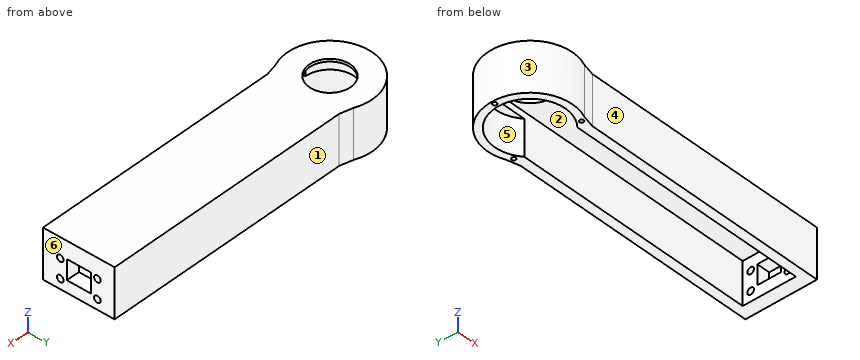
```python
from build123d import *

# Parameters (mm, degrees)
SKETCH025_R           = 32
PAD016_DEPTH          = 37
SKETCH026_R           = 18.5
POCKET001_DEPTH       = 35
SKETCH027_R           = 26.5
POCKET002_DEPTH       = 27
SKETCH028_R           = 15.5
POCKET003_DEPTH       = 37.001
PAD018_DEPTH          = 37
SKETCH034_W           = 40
SKETCH034_H           = 32
POCKET004_DEPTH       = 200
SKETCH046_W           = 54
SKETCH046_H           = 37
SKETCH046_W_2         = 18
SKETCH046_H_2         = 15
PAD020_DEPTH          = 10
SKETCH047_R           = 1.5
POCKET_DEPTH          = 10
POLARPATTERN003_COUNT = 3
CHAMFER002_SIZE       = 5
SKETCH063_R           = 2.5
POCKET022_DEPTH       = 10.001
BODY_PLACEMENT_ANGLE  = 179.999986


with BuildPart() as part:
    # Sketch025 (on Face1 of CopyPocket) → Pad016 (new body)
    with BuildSketch(Plane.XY.offset(19.5)):
        Circle(SKETCH025_R)
    extrude(amount=-PAD016_DEPTH)

    # Sketch026 (on Face3 of Pad016) → Pocket001 (cut)
    with BuildSketch(Plane(origin=(0, 0, -17.5), x_dir=(1, 0, 0), z_dir=(0, 0, -1))):
        Circle(SKETCH026_R)
    extrude(amount=-POCKET001_DEPTH, mode=Mode.SUBTRACT)

    # Sketch027 (on Face3 of Pocket001) → Pocket002 (cut)
    with BuildSketch(Plane(origin=(0, 0, -17.5), x_dir=(1, 0, 0), z_dir=(0, 0, -1))):
        Circle(SKETCH027_R)
    extrude(amount=-POCKET002_DEPTH, mode=Mode.SUBTRACT)

    # Sketch028 (on Face2 of Pocket002) → Pocket003 (cut, through all)
    with BuildSketch(Plane.XY.offset(19.5)):
        Circle(SKETCH028_R)
    extrude(amount=-POCKET003_DEPTH, mode=Mode.SUBTRACT)

    # Sketch030 (on Face2 of Pocket003) → Pad018 (join)
    with BuildSketch(Plane.XY.offset(19.5)):
        with BuildLine():
            ThreePointArc((-17.175564, 27), (-32, 0), (-17.175564, -27))
            Line((-200, -27), (-17.175564, -27))
            Line((-200, 27), (-200, -27))
            Line((-17.175564, 27), (-200, 27))
        make_face()
    extrude(amount=-PAD018_DEPTH)

    # Sketch034 (on Face2 of Pad018) → Pocket004 (cut)
    with BuildSketch(Plane(origin=(-200, 0, 0), x_dir=(0, -1, 0), z_dir=(-1, 0, 0))):
        with Locations((0, -1.5)):
            Rectangle(SKETCH034_W, SKETCH034_H)
    extrude(amount=-POCKET004_DEPTH, mode=Mode.SUBTRACT)

    # Sketch046 (on Face3 of Pocket004) → Pad020 (join)
    with BuildSketch(Plane(origin=(-200, 0, 0), x_dir=(0, -1, 0), z_dir=(-1, 0, 0))):
        with Locations((0, 1)):
            Rectangle(SKETCH046_W, SKETCH046_H)
        with Locations((0, -1)):
            Rectangle(SKETCH046_W_2, SKETCH046_H_2, mode=Mode.SUBTRACT)
    extrude(amount=PAD020_DEPTH)

    # Sketch047 (on Face20 of Pad020) → Pocket (cut)
    with BuildSketch(Plane(origin=(0, 0, -17.5), x_dir=(1, 0, 0), z_dir=(0, 0, -1))):
        with Locations((29.53, 0)):
            Circle(SKETCH047_R)
    pocket = extrude(amount=-POCKET_DEPTH, mode=Mode.SUBTRACT)

    # PolarPattern003: Pocket ×3 about axis
    polarpattern003_axis = Axis((0, 0, -17.5), (0, 0, -1))
    for i in range(1, POLARPATTERN003_COUNT):
        add(pocket.rotate(polarpattern003_axis, i * 360 / POLARPATTERN003_COUNT), mode=Mode.SUBTRACT)

    # Chamfer002
    chamfer002_edges = [part.edges().sort_by_distance(p)[0] for p in [
        (-17.175564, -27, 1),
        (-17.175564, 27, 1),
    ]]
    chamfer(chamfer002_edges, length=CHAMFER002_SIZE)

    # Sketch063 (on Face14 of Chamfer002) → Pocket022 (cut, through all)
    with BuildSketch(Plane.YZ.offset(-200)):
        with Locations((-14, 4.5)):
            Circle(SKETCH063_R)
        with Locations((14, 4.5)):
            Circle(SKETCH063_R)
        with Locations((-14, -10)):
            Circle(SKETCH063_R)
        with Locations((14, -10)):
            Circle(SKETCH063_R)
    extrude(amount=-POCKET022_DEPTH, mode=Mode.SUBTRACT)


with BuildPart() as part_1:
    # Body placement: moved
    add(part.part.moved(Location((5, -1e-06, 2.46221))).rotate(Axis((5, -1e-06, 2.46221), (0, 0, 1)), BODY_PLACEMENT_ANGLE))


solid = part_1.part
```
CAD build for the part. Positions are in the model's coordinates, mm. Face numbers are marked on the shaded views. A direction names the side the tool comes from. Give positions to 0.01 mm unless a question says otherwise; leave off trailing zeros. Write each loop counter-clockwise with the first axis right and the second up, starting at its lowest first coordinate (ties: lowest second). Pieces come first, ordered by that corner, then holes. Notation, with made-up numbers: M 54,57 L 113,57 A10 ccw 113,64 Z; hole C 54.5,-12 d3. An arc over 180 degrees is marked long. Return JSON: item names as keys, results as strings. Group by question number.
(1) Flat gauge pins, fed straight in: pin 1 Ø2 at (x, z) = (96.5, 14.5) entering from +Y; pin 2 Ø6 at (x, z) = (120.5, -7.5) entering from -Y; pin 3 Ø1.5 at (x, y) = (-24.5, 0.5) entering from -Z. Where does each tip first touch, or does it go through?
(2) 3-axis set-ups, long thin cutter, end or side, ignore diameter. For the marked faces 1, 2 and 3: which of +Z, -Z, +X, -X, +Y, -Y reach the whole face in a straight line?
(3) Mould opens along X. For the marked faces 4, 5 and 6 say: pulls with the +X half, pulls with the -X half, needs draft (parallel to the pull), parting line crosses it, or undercut.
(4) Band-saw the part on A-A (x = 103.5). Give the cut face in (y, z), and give its area (3 significant figures).
(5) Drill centre lines: L1, parallel to Y at x = 102.5, z = -8; L2, parallel to Y at x = 5, z = -9.25; L3, parallel to Z at x = 188.5, y = 5. Where is each one in solid material? Low to high. Write a range as [from, to].
Entries:
{
 "1": {"pin 1": "stops at y = 27", "pin 2": "stops at y = -27", "pin 3": "stops at z = -5.04"},
 "2": {"face 1": "+Z, -Z, +X, +Y", "face 2": "-Z", "face 3": "+Z, -Z"},
 "3": {"face 4": "needs draft", "face 5": "undercut", "face 6": "pulls with the +X half"},
 "4": {"outline": "M -27,-15.04 L -20,-15.04 L -20,16.96 L 20,16.96 L 20,-15.04 L 27,-15.04 L 27,21.96 L -27,21.96 Z", "area": "718 mm^2"},
 "5": {"L1": "y = [-27, -20], [20, 27]", "L2": "y = [-32, -26.5], [26.5, 32]", "L3": "z = [16.96, 21.96]"}
}
